Work out the finished part from the listing and answer in its coordinate system (mm). Coordinates: 2 decimals unless noted, no trailing zeros. Loops run counter-clockwise (first coordinate to the right, second up) from the corner with the lowest first, then second, coordinate; pieces in that order, holes last. Notation, with made-up numbers: (33.5, 55.5) -> (62.5, 55.5) arc R26 ccw to (62.5, 78.5) -> close; hole circle Ø6 at (52.25, 30.5). An arc over 180 degrees is marked (long way). One line per question, with ' | ' between items.
```python
from build123d import *

# Parameters (mm, degrees)
SKETCH1_W           = 64
SKETCH1_H           = 38
BOSS_EXTRUDE1_DEPTH = 1.57875
CHAMFER1_SIZE       = 2
SKETCH3_R           = 1.35
CUT_EXTRUDE1_DEPTH  = 38.249059741


with BuildPart() as part:
    # Sketch1 → Boss-Extrude1 (new body)
    with BuildSketch(Plane(origin=(0, 0, 0), x_dir=(1, 0, 0), z_dir=(0, 1, 0))):
        Rectangle(SKETCH1_W, SKETCH1_H)
    extrude(amount=BOSS_EXTRUDE1_DEPTH)

    # Chamfer1
    chamfer1_edges = [part.edges().sort_by_distance(p)[0] for p in [
        (32, 0.789375, 19),
        (-32, 0.789375, 19),
        (-32, 0.789375, -19),
        (32, 0.789375, -19),
    ]]
    chamfer(chamfer1_edges, length=CHAMFER1_SIZE)

    # Sketch3 → Cut-Extrude1 (cut, through all)
    with BuildSketch(Plane(origin=(0, 1.57875, 0), x_dir=(1, 0, 0), z_dir=(0, 1, 0))):
        with Locations(Location((-16.46, 15.5, 0), (0, 0, 270))):
            Circle(SKETCH3_R)
        with Locations(Location((16.46, 15.5, 0), (0, 0, 270))):
            Circle(SKETCH3_R)
        with Locations(Location((0, -15.5, 0), (0, 0, 270))):
            Circle(SKETCH3_R)
    extrude(amount=-CUT_EXTRUDE1_DEPTH, mode=Mode.SUBTRACT)


solid = part.part
```
1) The mould has two halves that part along X. Classify faces 1 (the face through (0, 0, 0)), 2 (the face through (31, 1, -18)), 3 (the face through (-17.78, 0.8, -15.79)): released by +X, released by -X, zero draft, split by the parting line, or undercut.
Check values:
face 1: zero draft | face 2: released by +X | face 3: undercut
2) Find section C-C (z = -16). Write down the section's boundary in (x, y), plus the area to 3 significant figures.
Check values:
outline: (-32, 0) -> (-17.71, 0) -> (-17.71, 1.58) -> (-32, 1.58) -> close; (-15.21, 0) -> (15.21, 0) -> (15.21, 1.58) -> (-15.21, 1.58) -> close; (17.71, 0) -> (32, 0) -> (32, 1.58) -> (17.71, 1.58) -> close | area: 93.1 mm^2
3) Find section B-B (x = -16.46). Write down the section's boundary in (y, z), plus the area to 3 significant figures.
Check values:
outline: (0, -19) -> (1.58, -19) -> (1.58, -16.85) -> (0, -16.85) -> close; (0, -14.15) -> (1.58, -14.15) -> (1.58, 19) -> (0, 19) -> close | area: 55.7 mm^2
4) Find the intervals of material crossed by line 1 along X through (y, z) = (1.2, -15.5); line 2 along Z through (x, y) = (16.5, 1.2); line 3 along X through (y, z) = (0.9, 15.5), in increasing order.
Check values:
line 1: x = -32 to -17.81, -15.11 to 15.11, 17.81 to 32 | line 2: z = -19 to -16.85, -14.15 to 19 | line 3: x = -32 to -1.35, 1.35 to 32
5) Find section A-A (z = 15.5). Write down the section's boundary in (x, y).
Check values:
outline: (-32, 0) -> (-1.35, 0) -> (-1.35, 1.58) -> (-32, 1.58) -> close; (1.35, 0) -> (32, 0) -> (32, 1.58) -> (1.35, 1.58) -> close
